Geometry check sheet. Reference: the model listing, model coordinates, mm. A direction names the side the tool comes from. Coordinates: 2 decimals unless noted, no trailing zeros. Order: outer loops, then holes, each group sorted by start corner. A loop starts at its lowest first (then second) coordinate and runs counter-clockwise, first axis right, second up. Notation, with made-up numbers: (2, 51.5) - (24, 51.5) arc R19 cw to (24, 62.5) - close; hole circle Ø3 at (39, -5.5). An arc over 180 degrees is marked (long way). One line per item, written item: value. Start each with the question number.
Autodesk Inventor part; units mm, degrees
ref_plane "Start Plane" through (0, 0, 30) normal (0, 0, 1) x (1, 0, 0)
ref_plane "End Plane" through (0, 0, 2000) normal (0, 0, 1) x (1, 0, 0)
ref_plane "Work Plane4" through (-1750, -22, 30) normal (0, 0, -1) x (-1, 0, 0)
ref_plane "Start Plane" through (0, 0, 30) normal (0, 0, 1) x (1, 0, 0)
ref_plane "End Plane" through (0, 0, 2000) normal (0, 0, 1) x (1, 0, 0)
sketch "Sketch" plane through (0, 0, 0) normal (0, 0, 1) x (1, 0, 0)
  line L0 (-30, -22) -> (-30, 22)
  line L1 (-22, 30) -> (22, 30)
  line L2 (30, 22) -> (30, -22)
  line L3 (22, -30) -> (-22, -30)
  arc A0 (-30, -22) -> (-22, -30) centre (-22, -22) ccw
  arc A1 (30, 22) -> (22, 30) centre (22, 22) ccw
  arc A2 (-22, 30) -> (-30, 22) centre (-22, 22) ccw
  arc A3 (22, -30) -> (30, -22) centre (22, -22) ccw
  arc A4 (-22, 26) -> (-26, 22) centre (-22, 22) ccw
  line L4 (-22, 26) -> (22, 26)
  arc A5 (26, 22) -> (22, 26) centre (22, 22) ccw
  line L5 (26, 22) -> (26, -22)
  arc A6 (22, -26) -> (26, -22) centre (22, -22) ccw
  line L6 (22, -26) -> (-22, -26)
  arc A7 (-26, -22) -> (-22, -26) centre (-22, -22) ccw
  line L7 (-26, -22) -> (-26, 22)
  line L8 (0, 44.3196) -> (0, -44.3196) construction
  line L9 (-44.3196, 0) -> (44.3196, 0) construction
  dimension "d7" = 8
  dimension "d9" = 60
  dimension "d11" = 60
  dimension "d12" = 4
  dimension "d15" = 30
  dimension "d16" = 30
extrude "Body" add sketch "Sketch" along normal up to surface (1970 mm away) from surface at 30
sketch "Sketch3" plane through (0, 0, 0) normal (0, 0, 1) x (1, 0, 0)
  line L0 (0, 0) -> (10, 0)
ref_plane "Work Plane3" through (0, 0, 0) normal (0, -1, 0) x (1, 0, 0)
ref_plane "Work Plane4" through (-1750, -22, 30) normal (0, 0, -1) x (-1, 0, 0)
split "Split1" plane through (-1750, -22, 30) removes the side toward (0, 0, -1)
sketch "Sketch4" plane through (0, 0, 0) normal (0, -1, 0) x (1, 0, 0)
  line L0 (-2, 30) -> (12, 30)
  line L1 (-2, 2000) -> (12, 2000)
  dimension "d18" = 1970
equation "\"d7\" = G_IR"
equation "\"d9\" = G_W"
equation "\"d11\" = G_H"
equation "\"d12\" = G_T"
equation "\"d15\" = 0.5 * d9"
equation "\"d16\" = 0.5 * d11"
equation "\"d3\" = G_L"
equation "\"G_W\" = 60"
equation "\"G_H\" = 60"
equation "\"G_T\" = 4"
equation "\"G_IR\" = 8"
equation "\"G_L\" = d18"
equation "\"G_OFFSET_END\" = 0"
properties part number "ISO 10799-2 - 60x60x4 - 1970" material "Steel, Mild"
Q1. Material ranges on probe 1 along X at (y, z) = (-4.5, 1668); probe 2 along X at (y, z) = (-23.5, 836), recorded low to high.
Q2. Cross-section at B-B, the plane z = 481.5. Enter the section's corners in (x, y), and give its area (3 significant figures).
Q3. Gauge pin test, flat end, axial feed: P1, Ø8, axis at x = 19.5, y = 12, coming from the +Z side. Record the tip position at first contact, or that the pin passes through.
Q4. Cross-section at A-A, the plane y = -6. Enter the section's corners in (x, z), and give its area (3 significant figures).
Q5. Set-up check for faces 1 (the flat face through (-27, 0, 30)), 2 (the flat face through (0, -26, 1001)): record each of +Z, -Z, +X, -X, +Y, -Y from which the full face is reachable in a straight line by a thin tool's end or side.
Q6. Release check for a two-part mould opening along Y. For faces 3 (the flat face through (-27, 0, 2000)), 4 (the flat face through (0, 30, 1001)), 5 (the flat face through (0, 26, 1001)) record: released by +Y, released by -Y, zero draft, split by the parting line, or undercut.
Check result:
1. probe 1: x = -30 to -26, 26 to 30
1. probe 2: x = -29.86 to -25.71, 25.71 to 29.86
2. outline: (-30, -22) arc R8 ccw to (-22, -30) - (22, -30) arc R8 ccw to (30, -22) - (30, 22) arc R8 ccw to (22, 30) - (-22, 30) arc R8 ccw to (-30, 22) - close; hole (-26, -22) arc R4 ccw to (-22, -26) - (22, -26) arc R4 ccw to (26, -22) - (26, 22) arc R4 ccw to (22, 26) - (-22, 26) arc R4 ccw to (-26, 22) - close
2. area: 855 mm2
3. P1: passes through
4. outline: (-30, 30) - (-26, 30) - (-26, 2000) - (-30, 2000) - close; (26, 30) - (30, 30) - (30, 2000) - (26, 2000) - close
4. area: 15,800 mm2
5. face 1: -Z, +X, -X, +Y, -Y
5. face 2: +Z, -Z
6. face 3: zero draft
6. face 4: released by +Y
6. face 5: undercut
